from build123d import *

# Parameters (mm, degrees)
F0_W     = 136.9216442108
F0_H     = 85.8872830868
F1_DEPTH = 12.7
F3_DEPTH = 63.5
F4_R     = 38.1241365852
F5_DEPTH = 63.5
F6_W     = 56.9095164537
F6_H     = 13.9519274235
F7_DEPTH = 44.45
F9_DEPTH = 25.4


with BuildPart() as f1:
    # F0 (on Top) → F1 (new body)
    with BuildSketch(Plane.XY):
        Rectangle(F0_W, F0_H)
    extrude(amount=F1_DEPTH)

    # F2 (on face) → F3 (join)
    with BuildSketch(Plane.XY.offset(12.7)):
        with BuildLine():
            ThreePointArc((32.8620942883, -42.9436415434), (84.2442332892, -44.2877306594), (110.3311590742, 0))
            ThreePointArc((110.3311590742, 0), (84.2442332892, 44.2877306594), (32.8620942883, 42.9436415434))
            Line((32.8620942883, 42.9436415434), (68.4608221054, 42.9436415434))
            Line((68.4608221054, 42.9436415434), (68.4608221054, -42.9436415434))
            Line((68.4608221054, -42.9436415434), (32.8620942883, -42.9436415434))
        make_face()
        with BuildLine():
            Line((68.4608221054, 42.9436415434), (32.8620942883, 42.9436415434))
            ThreePointArc((32.8620942883, 42.9436415434), (9.0570263673, 0), (32.8620942883, -42.9436415434))
            Line((32.8620942883, -42.9436415434), (68.4608221054, -42.9436415434))
            Line((68.4608221054, -42.9436415434), (68.4608221054, 42.9436415434))
        make_face()
    extrude(amount=F3_DEPTH)

    # F4 (on face) → F5 (cut)
    with BuildSketch(Plane.XY.offset(76.2)):
        with Locations((59.6940927207, 0)):
            Circle(F4_R)
    extrude(amount=-F5_DEPTH, mode=Mode.SUBTRACT)

    # F6 (on face) → F7 (join)
    with BuildSketch(Plane.XY.offset(12.7)):
        with Locations((-19.1295444965, 0)):
            Rectangle(F6_W, F6_H)
    extrude(amount=F7_DEPTH)

    # F8 (on face) → F9 (cut)
    with BuildSketch(Plane(origin=(0, 6.9759637117, 0), x_dir=(-1, 0, 0), z_dir=(0, 1, 0))):
        Polygon((47.5843027234, 57.15), (-9.3252137303, 57.15), (47.5843027234, 12.7), align=None)
    extrude(amount=-F9_DEPTH, mode=Mode.SUBTRACT)


solid = f1.part
Here's how the part is built. I have some questions about the finished solid (model axes, mm). A direction names the side the tool comes from. Give positions to 0.01 mm unless a question says otherwise; leave off trailing zeros. Order: outer loops, then holes, each group sorted by start corner. A loop starts at its lowest first (then second) coordinate and runs counter-clockwise, first axis right, second up. Notation, with made-up numbers: M 43,18 L 91,18 A13 ccw 91,33 Z; hole C 10,44.5 d9. An arc over 180 degrees is marked long. Answer as a JSON object with one key per item and string values. Group by question number.
1) We'd pull the mould along Y, two halves only. Please class faces 5 (the flat face through (50, 1, 12.7)), 6 (the flat face through (-30, 10, 12.7)), 7 (the flat face through (-1, -42.944, 6)): pulls with the +Y half, pulls with the -Y half, needs draft (parallel to the pull), parting line crosses it, or undercut.
2) Suppose I cut it at D-D, the plane x = -12.5. Write out the boundary of the cut face in (y, z), plus the area to 3 significant figures.
3) Please list where these lines run through material, in increasing order: L1, parallel to Z at x = 11.5, y = 19; L2, parallel to X at y = 17, z = 59; L3, parallel to X at y = -3, z = 40. Write a range as [from, to].
4) Suppose I cut it at A-A, the plane y = 0. Write out the boundary of the cut face in (x, z), plus the area to 3 significant figures.
5) Suppose I cut it at C-C, the plane z = 66. Write out the boundary of the cut face in (x, y), plus the area to 3 significant figures.
6) I'm going to push flat-ended pins straight in: pin 1 Ø6 at (y, z) = (-19, 62.5) entering from -X; pin 2 Ø12 at (y, z) = (7.5, 18) entering from +X; pin 3 Ø14 at (y, z) = (-7, 3.5) entering from +X. Where does each tip first touch, or does it pass through?
7) On a 3-axis mill with a long thin cutter (end or side, diameter ignored), from which of +Z, -Z, +X, -X, +Y, -Y can I reach the whole of each face in a straight line? I mean faces 1 (the flat face through (68.461, -1, 6)), 2 (the cylindrical face through (29.44, -23.2, 44.89)), 3 (the flat face through (-1, 42.944, 6)), 4 (the flat face through (-7, 6.976, 25)). Say none if no direction works.
8) Suppose I cut it at B-B, the plane x = 73. Write out the boundary of the cut face in (y, z), plus the area to 3 significant figures.
Results found:
{
 "1": {"face 5": "undercut", "face 6": "needs draft", "face 7": "pulls with the -Y half"},
 "2": {"outline": "M -42.94,0 L 42.94,0 L 42.94,12.7 L 6.98,12.7 L 6.98,40.1 L -6.98,40.1 L -6.98,12.7 L -42.94,12.7 Z", "area": "1,470 mm²"},
 "3": {"L1": "[0, 12.7]", "L2": "[12, 25.57], [93.82, 107.39]", "L3": "[-12.63, 21.69], [97.7, 110.24]"},
 "4": {"outline": "M -68.46,0 L 68.46,0 L 68.46,12.7 L 21.57,12.7 L 21.57,76.2 L 9.06,76.2 L 9.06,57.15 L 9.33,57.15 L -47.58,12.7 L -68.46,12.7 Z; M 97.82,12.7 L 110.33,12.7 L 110.33,76.2 L 97.82,76.2 Z", "area": "4,580 mm²"},
 "5": {"outline": "C 59.69,0 d101.27; hole C 59.69,0 d76.25", "area": "3,490 mm²"},
 "6": {"pin 1": "x = 11.65", "pin 2": "x = 110.31", "pin 3": "x = 68.46"},
 "7": {"face 1": "-Z, +X, +Y, -Y", "face 2": "+Z", "face 3": "-Z, +X, -X, +Y", "face 4": "+Z, -X, +Y"},
 "8": {"outline": "M -48.86,12.7 L -35.73,12.7 L -35.73,76.2 L -48.86,76.2 Z; M 35.73,12.7 L 48.86,12.7 L 48.86,76.2 L 35.73,76.2 Z", "area": "1,670 mm²"}
}
